The drawing under review shows one solid part. Ordinate dimensions are in mm from its lowest x, y, z. A direction names the side the tool comes from. Round coordinates to 2 decimals unless told otherwise and drop trailing zeros. Write each loop counter-clockwise with the first axis right and the second up, starting at its lowest first coordinate (ties: lowest second). Pieces come first, ordered by that corner, then holes. Notation, with made-up numbers: M 1.25,9 L 44.25,9 A11 ccw 44.25,19 Z; hole C 3,24.25 d8. An arc over 180 degrees is marked long. One line per item, written item: value. Start each with the question number.
1) Tool access review of the marked faces 4, 5 and 6: name each direction out of +Z, -Z, +X, -X, +Y, -Y from which nothing blocks a thin tool from reaching the whole face with its end or side.
2) Take a section at D-D, the plane y = 6.5. Write out the cut boundary in (x, z), and give its area (3 significant figures).
3) Take a section at A-A, the plane z = 10. State how many separate pieces and enclosed holes the cut face has, and give its area (3 significant figures).
4) For P1, Ø8, axis at y = 9.5, z = 7.5, coming from the -X side; P2, Ø2, axis at y = 29.5, z = 3.5, coming from the -X side; P3, Ø4.5, axis at x = 4.5, z = 12, coming from the -Y side, all flat-tipped, find the tip position at first contact; note any pin that passes through.
5) Wall thickness on probe 1 along Z at (x, y) = (6, 34.45); probe 2 along Y at (x, z) = (3, 1.5); probe 3 along Y at (x, z) = (14.5, 12.75): over which ranges is each line inside the solid? List them lowest first.
6) Take a section at B-B, the plane x = 6. Write out the cut boundary in (y, z).
7) Mouldability with a two-part tool opening along X and no side actions: class the marked faces 1, 2 and 3 as +X half, -X half, draft (parallel to the pull), parting line (faces both ways), or undercut.
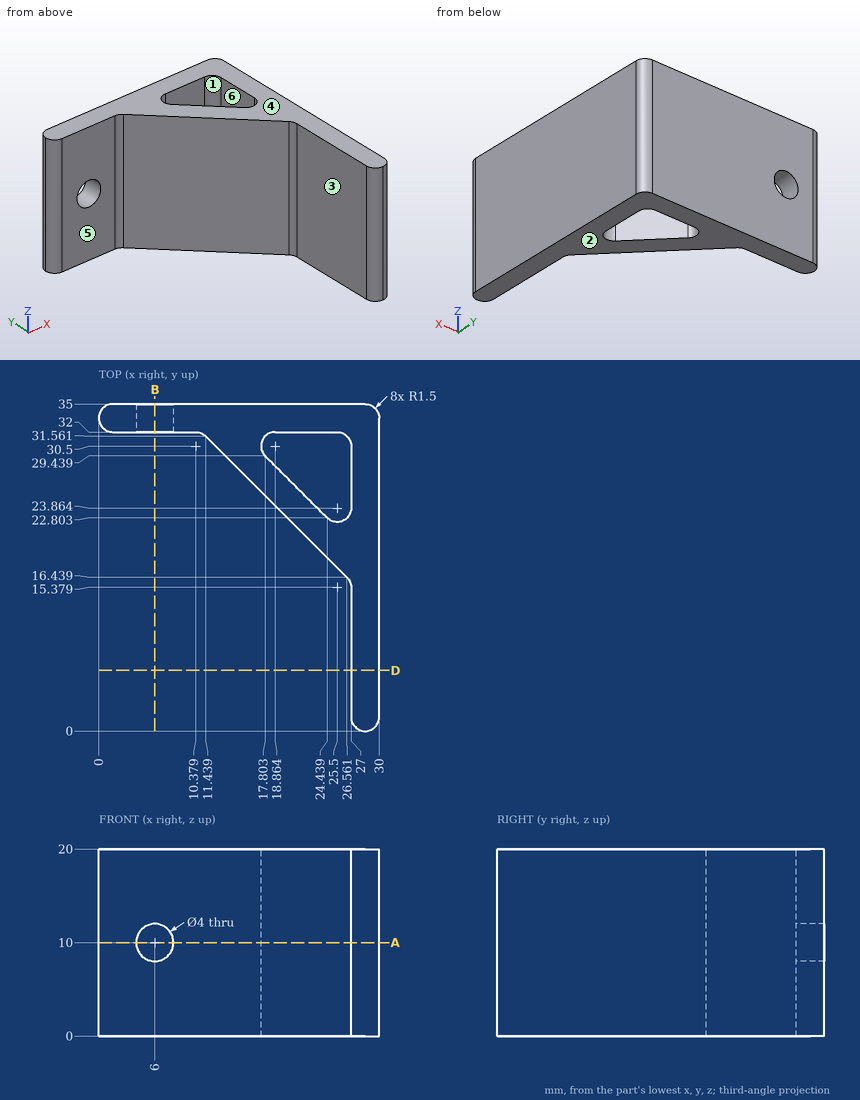
Checked values:
1. face 4: +Z, +X, -X, +Y, -Y
1. face 5: +Z, -Z, -X, -Y
1. face 6: +Z, -Z
2. outline: M 27,0 L 30,0 L 30,20 L 27,20 Z
2. area: 60.0 mm2
3. separate pieces: 2
3. enclosed holes: 1
3. area: 237 mm2
4. P1: stops at x = 27
4. P2: stops at x = 12.5
4. P3: stops at y = 32
5. probe 1: z = 0 to 8, 12 to 20
5. probe 2: y = 32 to 35
5. probe 3: y = 28.5 to 35
6. outline: M 32,0 L 35,0 L 35,8 L 32,8 Z; M 32,12 L 35,12 L 35,20 L 32,20 Z
7. face 1: undercut
7. face 2: draft
7. face 3: -X half
